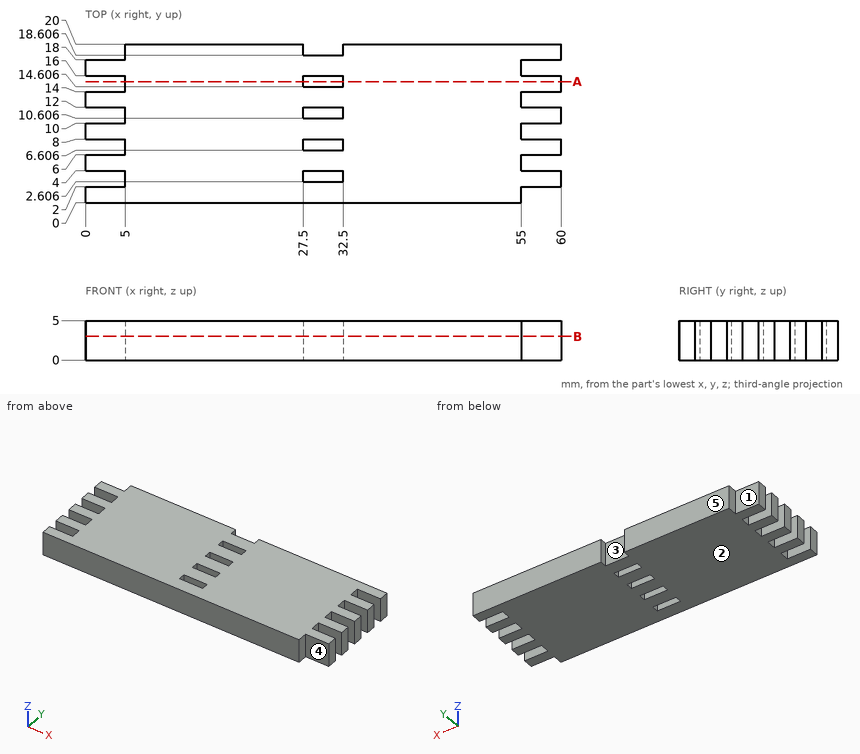
Verification items for this drawing (mm, ordinates from the low corner). A direction names the side the tool comes from. Round coordinates to 2 decimals unless told otherwise and drop trailing zeros. Write each loop counter-clockwise with the first axis right and the second up, starting at its lowest first coordinate (ties: lowest second). Pieces come first, ordered by that corner, then holes. Notation, with made-up numbers: M 5.5,80.25 L 52.5,80.25 A15 cw 52.5,102.25 Z; hole C 6.25,29 d2. An arc over 180 degrees is marked long. Write item = value, one per line. Start each with the question number.
1. Section check A-A, the plane y = 15.25. Record the cut outline in (x, z).
2. Section check B-B, the plane z = 3. State how many separate pieces and enclosed holes the cut face has, then the cut area to 4 significant figures.
3. Tool access check on the marked faces 1, 2, 3, 4 and 5. Record the directions out of +Z, -Z, +X, -X, +Y, -Y that give a thin tool (end or side, any length) a straight path to the whole face; none if there is none.
4. Gauge pin test, flat end, axial feed: pin 1 (1.5 mm diameter, centred on y = 19.5, z = 1.5, fed in from -X). Record the tip position at first contact, or that the pin passes through.
5. Scan lines: line 1 (Y direction, x = 30, z = 3.85); line 2 (Y direction, x = 55.5, z = 2.8); line 3 (X direction, y = 18.75, z = 0.65). Record each from-to range of solid material in increasing order. Write a range as [from, to].
Results found:
q1.outline = M 5,0 L 27.5,0 L 27.5,5 L 5,5 Z; M 32.5,0 L 60,0 L 60,5 L 32.5,5 Z
q2.separate_pieces = 1
q2.enclosed_holes = 4
q2.area = 1,065 mm^2
q3.face_1 = +Z, -Z, -X, +Y
q3.face_2 = -Z, +X, -X, +Y, -Y
q3.face_3 = +Z, -Z, +Y
q3.face_4 = +Z, -Z, +X, -Y
q3.face_5 = +Z, -Z, +X, -X, +Y
q4.pin_1 = 5
q5.line_1 = [0, 2.61], [4, 6.61], [8, 10.61], [12, 14.61], [16, 18.61]
q5.line_2 = [2, 4], [6, 8], [10, 12], [14, 16], [18, 20]
q5.line_3 = [5, 27.5], [32.5, 60]
